The model under review builds one solid part; all positions refer to its coordinate system, in mm. A direction names the side the tool comes from. Coordinates: 2 decimals unless noted, no trailing zeros. Use CSV: the item, a comma, the result in double quotes. Start each with the question number.
1. Draft analysis for pull direction X (two halves, no side actions). For faces 3 (the flat face through (-28, 100, 0)), 4 (the cylindrical face through (-5.077, -38.668, -14.465)), 5 (the cylindrical face through (-26.501, -119.343, -0.246)), state which applies: +X half, -X half, draft (parallel to the pull), parting line (faces both ways), or undercut.
2. For L1, parallel to Y at x = 0, z = -7.75; L2, parallel to X at y = 80, z = -8.5; L3, parallel to Y at x = -45.5, z = -1.5, list the stretches that pass through material, from the lowest coordinate up.
3. Tool access review of faces 1 (the cylindrical face through (-30.837, -138.867, -0.246)), 2 (the cylindrical face through (190.764, 60.075, -5.93)): name each direction out of +Z, -Z, +X, -X, +Y, -Y from which nothing blocks a thin tool from reaching the whole face with its end or side.
4. Clearance check with flat-ended pins moving along their axes: P1, Ø4, axis at y = -88.5, z = -3, coming from the +X side; P2, Ø6, axis at x = 150.5, z = -13.5, coming from the -Y side; P3, Ø6, axis at x = -133.5, y = 133.5, coming from the -Z side. State where each tip first meets the part, or that it passes through.
from build123d import *

# Parameters (mm, degrees)
F0_R      = 200
F1_DEPTH  = 12
F2_SIZE   = 1
F3_R      = 39
F4_DEPTH  = 6
F5_R      = 25
F6_DEPTH  = 25
F7_SIZE   = 1
F8_R      = 182.75
F8_R_2    = 182.25
F8_R_3    = 162.75
F8_R_4    = 162.25
F8_R_5    = 142.75
F8_R_6    = 142.25
F8_R_7    = 122.75
F8_R_8    = 122.25
F8_R_9    = 102.75
F8_R_10   = 102.25
F8_R_11   = 82.75
F8_R_12   = 82.25
F8_R_13   = 62.75
F8_R_14   = 62.25
F9_DEPTH  = 0.5
F10_R     = 4
F11_DEPTH = 25
F12_R     = 2.1
F13_DEPTH = 25
F12_R_2   = 4
F14_DEPTH = 4
F12_R_3   = 2.5
F15_DEPTH = 10
F12_R_4   = 1.5
F16_DEPTH = 6
F17_DEPTH = 25


with BuildPart() as f1:
    # F0 (on Top) → F1 (new body)
    with BuildSketch(Plane.XY):
        Circle(F0_R)
    extrude(amount=-F1_DEPTH)

    # F2
    f2_edges = [f1.edges().sort_by_distance(p)[0] for p in [
        (-200, 0, -12),
        (-200, 0, 0),
    ]]
    chamfer(f2_edges, length=F2_SIZE)

    # F3 (on face) → F4 (join)
    with BuildSketch(Plane(origin=(0, 0, -12), x_dir=(1, 0, 0), z_dir=(0, 0, -1))):
        Circle(F3_R)
    extrude(amount=F4_DEPTH)

    # F5 (on face) → F6 (cut)
    with BuildSketch(Plane.XY):
        Circle(F5_R)
    extrude(amount=-F6_DEPTH, mode=Mode.SUBTRACT)

    # F7
    f7_edges = [f1.edges().sort_by_distance(p)[0] for p in [
        (-39, 0, -18),
    ]]
    chamfer(f7_edges, length=F7_SIZE)

    # F8 (on face) → F9 (cut)
    with BuildSketch(Plane.XY):
        Circle(F8_R)
        Circle(F8_R_2, mode=Mode.SUBTRACT)
        Circle(F8_R_3)
        Circle(F8_R_4, mode=Mode.SUBTRACT)
        Circle(F8_R_5)
        Circle(F8_R_6, mode=Mode.SUBTRACT)
        Circle(F8_R_7)
        Circle(F8_R_8, mode=Mode.SUBTRACT)
        Circle(F8_R_9)
        Circle(F8_R_10, mode=Mode.SUBTRACT)
        Circle(F8_R_11)
        Circle(F8_R_12, mode=Mode.SUBTRACT)
        Circle(F8_R_13)
        Circle(F8_R_14, mode=Mode.SUBTRACT)
    extrude(amount=-F9_DEPTH, mode=Mode.SUBTRACT)

    # F10 (on face) → F11 (cut)
    with BuildSketch(Plane.XY):
        with Locations((90, 0)):
            Circle(F10_R)
        with Locations((45, 77.9422863406)):
            Circle(F10_R)
        with Locations((-45, 77.9422863406)):
            Circle(F10_R)
        with Locations((-90, 0)):
            Circle(F10_R)
        with Locations((-45, -77.9422863406)):
            Circle(F10_R)
        with Locations((45, -77.9422863406)):
            Circle(F10_R)
    extrude(amount=-F11_DEPTH, mode=Mode.SUBTRACT)

    # F12 (on face) → F13 (cut)
    with BuildSketch(Plane.XY):
        with Locations((-43.75, 0)):
            Circle(F12_R)
        with Locations((0, 43.75)):
            Circle(F12_R)
        with Locations((43.75, 0)):
            Circle(F12_R)
        with Locations((0, -43.75)):
            Circle(F12_R)
    extrude(amount=-F13_DEPTH, mode=Mode.SUBTRACT)

    # F12 (on face) → F14 (cut)
    with BuildSketch(Plane.XY):
        with Locations((-43.75, 0)):
            Circle(F12_R_2)
        with Locations((-43.75, 0)):
            Circle(F12_R, mode=Mode.SUBTRACT)
        with Locations((0, -43.75)):
            Circle(F12_R_2)
        with Locations((0, -43.75)):
            Circle(F12_R, mode=Mode.SUBTRACT)
        with Locations((43.75, 0)):
            Circle(F12_R_2)
        with Locations((43.75, 0)):
            Circle(F12_R, mode=Mode.SUBTRACT)
        with Locations((0, 43.75)):
            Circle(F12_R_2)
        with Locations((0, 43.75)):
            Circle(F12_R, mode=Mode.SUBTRACT)
    extrude(amount=-F14_DEPTH, mode=Mode.SUBTRACT)

    # F12 (on face) → F15 (cut)
    with BuildSketch(Plane.XY):
        with Locations((-21.2132034356, 21.2132034356)):
            Circle(F12_R_3)
        with Locations((21.2132034356, 21.2132034356)):
            Circle(F12_R_3)
        with Locations((-21.2132034356, -21.2132034356)):
            Circle(F12_R_3)
        with Locations((21.2132034356, -21.2132034356)):
            Circle(F12_R_3)
    extrude(amount=-F15_DEPTH, mode=Mode.SUBTRACT)

    # F12 (on face) → F16 (cut)
    with BuildSketch(Plane.XY):
        with Locations((0, -28.5)):
            Circle(F12_R_4)
        with Locations((28.5, 0)):
            Circle(F12_R_4)
        with Locations((-28.5, 0)):
            Circle(F12_R_4)
        with Locations((0, 28.5)):
            Circle(F12_R_4)
    extrude(amount=-F16_DEPTH, mode=Mode.SUBTRACT)

    # F12 (on face) → F17 (cut)
    with BuildSketch(Plane.XY):
        with Locations((13.3124752448, 28.5486952917)):
            Circle(F12_R_2)
        with Locations((-13.3124752448, -28.5486952917)):
            Circle(F12_R_2)
    extrude(amount=-F17_DEPTH, mode=Mode.SUBTRACT)


solid = f1.part
Computed:
1,face 3,"draft"
1,face 4,"parting line"
1,face 5,"undercut"
2,L1,"y = -200 to -45.85, -41.65 to -25, 25 to 41.65, 45.85 to 200"
2,L2,"x = -183.3 to -48.43, -41.57 to 41.57, 48.43 to 183.3"
2,L3,"y = -194.76 to -81.91, -73.97 to -3.6, 3.6 to 73.97, 81.91 to 194.76"
3,face 1,"+Z"
3,face 2,"+Z, -Z"
4,P1,"stops at x = 180.33"
4,P2,"stops at y = -133.6"
4,P3,"stops at z = -12"
